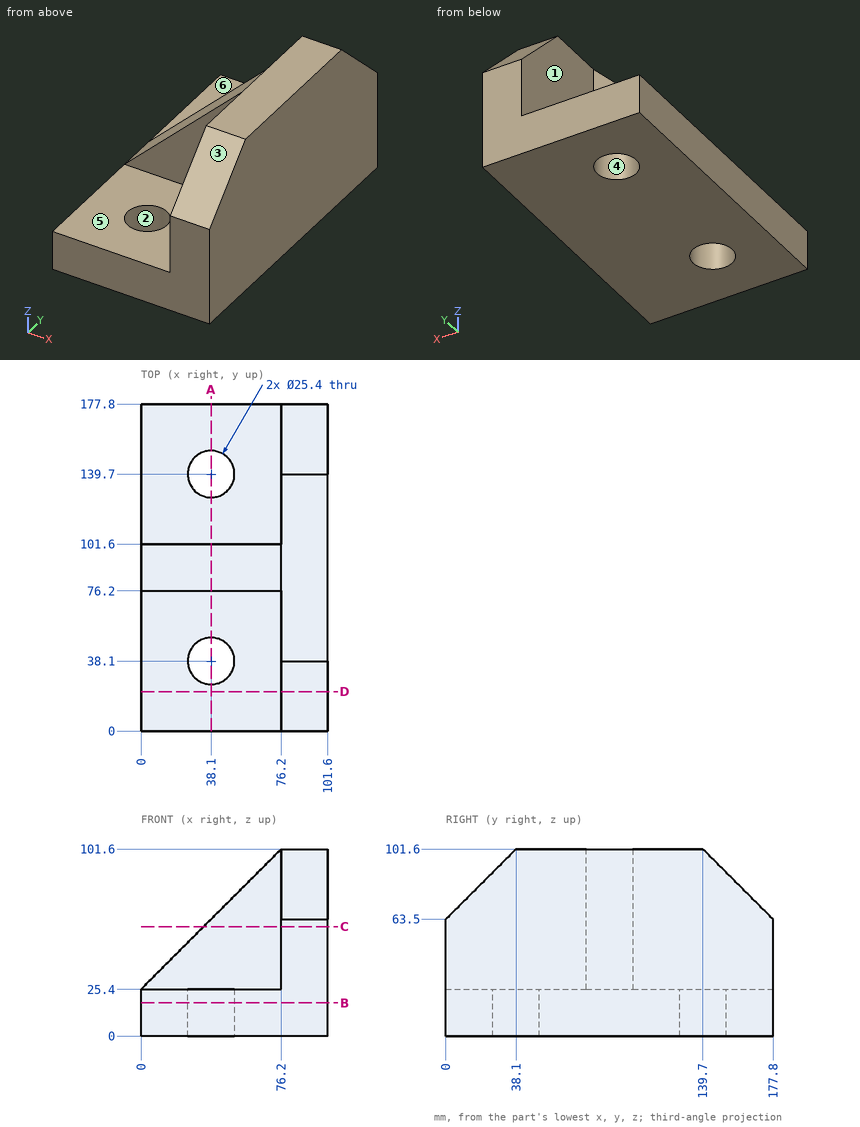
For this review, use the dimensioned drawing (mm, ordinates from the lowest corner) and the shaded views. A direction names the side the tool comes from. Round coordinates to 2 decimals unless told otherwise and drop trailing zeros. Write each loop counter-clockwise with the first axis right and the second up, starting at its lowest first coordinate (ties: lowest second). Pieces come first, ordered by that corner, then holes. Notation, with made-up numbers: (59.25, -29) - (68.25, -29) arc R25 ccw to (68.25, 10) - close; hole circle Ø8 at (31, -8). An arc over 180 degrees is marked (long way). Answer as CSV lines item,"result". Start each with the question number.
(1) Draft analysis for pull direction X (two halves, no side actions). For the marked faces 1, 2 and 3, state which applies: pulls with the +X half, pulls with the -X half, needs draft (parallel to the pull), parting line crosses it, or undercut.
(2) We need section D-D on y = 21.5. State the section outline as (x, z) points, plus the area to 3 significant figures.
(3) To check wall thickness, follow line 1 (Y direction, x = 38, z = 9); line 2 (X direction, y = 139, z = 12); line 3 (Y direction, x = 58, z = 64). State the ranges of each line that lie inside material, in increasing order.
(4) We need section C-C on z = 59.5. State the section outline as (x, y) points, plus the area to 3 significant figures.
(5) We need section B-B on z = 18. State the section outline as (x, y) points.
(6) We need section A-A on x = 38.1. State the section outline as (y, z) points, plus the area to 3 significant figures.
(7) For the marked faces 4, 5 and 6, list the 3-axis set-ups (+Z, -Z, +X, -X, +Y, -Y) from which the entire face can be reached by the end or side of a thin tool; tool diameter is ignored.
(8) For pin 1 Ø10 at (x, z) = (15, 39.5) entering from +Y, flat-tipped, find the tip position at first contact; note if it passes through.
Worked answers:
1,face 1,"pulls with the -X half"
1,face 2,"undercut"
1,face 3,"needs draft"
2,outline,"(0, 0) - (101.6, 0) - (101.6, 85) - (76.2, 85) - (76.2, 25.4) - (0, 25.4) - close"
2,area,"4,090 mm²"
3,line 1,"0 to 25.4, 50.8 to 127, 152.4 to 177.8"
3,line 2,"0 to 25.42, 50.78 to 101.6"
3,line 3,"76.2 to 101.6"
4,outline,"(34.1, 76.2) - (76.2, 76.2) - (76.2, 0) - (101.6, 0) - (101.6, 177.8) - (76.2, 177.8) - (76.2, 101.6) - (34.1, 101.6) - close"
4,area,"5,590 mm²"
5,outline,"(0, 0) - (101.6, 0) - (101.6, 177.8) - (0, 177.8) - close; hole circle Ø25.4 at (38.1, 38.1); hole circle Ø25.4 at (38.1, 139.7)"
6,outline,"(0, 0) - (25.4, 0) - (25.4, 25.4) - (0, 25.4) - close; (50.8, 0) - (127, 0) - (127, 25.4) - (101.6, 25.4) - (101.6, 63.5) - (76.2, 63.5) - (76.2, 25.4) - (50.8, 25.4) - close; (152.4, 0) - (177.8, 0) - (177.8, 25.4) - (152.4, 25.4) - close"
6,area,"4,190 mm²"
7,face 4,"+Z, -Z"
7,face 5,"+Z, -X, -Y"
7,face 6,"+Z, -X, +Y"
8,pin 1,"y = 101.6"
